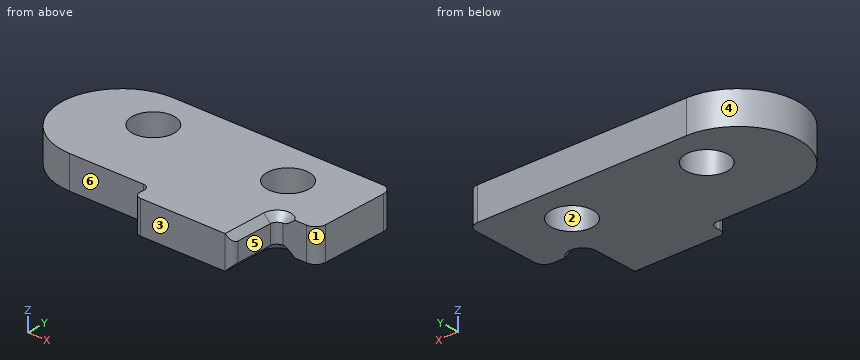
```python
from build123d import *

# Parameters (mm, degrees)
CROQUIS1_R                       = 6.125
SALIENTE_EXTRUIR1_DEPTH          = 9.53
BRIDA_DE_ARISTA1_STRIP_W         = 57.18
BRIDA_DE_ARISTA1_STRIP_H         = 9.53
BRIDA_DE_ARISTA1_STRIP_CUT_DEPTH = 85
BRIDA_DE_ARISTA1_DEPTH           = 85
REDONDEO1_R                      = 10
CHAFL_N1_SIZE                    = 25
CHAFL_N1_SIZE2                   = 20
REDONDEO2_R                      = 20
CORTAR_EXTRUIR3_DEPTH            = 148.009594705
CORTAR_EXTRUIR3_DEPTH_BACK       = 148.009594705
CROQUIS7_W                       = 70
CROQUIS7_H                       = 50
CORTAR_EXTRUIR5_DEPTH            = 92.169188443
CORTAR_EXTRUIR5_DEPTH_BACK       = 92.169188443
CROQUIS8_W                       = 21.963248134
CROQUIS8_H                       = 19.06
CORTAR_EXTRUIR6_REACH            = 68.882
CROQUIS10_W                      = 12
CROQUIS10_H                      = 15
SALIENTE_EXTRUIR3_START          = -9.53
SALIENTE_EXTRUIR3_DEPTH          = 9.53
REDONDEO3_R                      = 3
REDONDEO4_R                      = 2
CHAFL_N2_SIZE                    = 2


# Sheet-metal steps are written as plain solids
with BuildPart() as part:
    # Croquis1 → Saliente-Extruir1 (new body)
    with BuildSketch(Plane.XY):
        with BuildLine():
            Line((-5, 12.5), (59.758688568, 12.5))
            ThreePointArc((59.758688568, 12.5), (63.068757982, 11.936283192), (66.005639043, 10.308688094))
            Line((66.005639043, 10.308688094), (70.527359279, 6.691311906))
            ThreePointArc((70.527359279, 6.691311906), (73.464240341, 5.063716808), (76.774309755, 4.5))
            Line((76.774309755, 4.5), (123.266499161, 4.5))
            ThreePointArc((123.266499161, 4.5), (125.848488059, 3.781744193), (127.688665549, 1.833333333))
            ThreePointArc((127.688665549, 1.833333333), (129.41356885, -2.692366017), (130, -7.5))
            Line((130, -7.5), (130, -37.5))
            Line((130, -37.5), (45, -37.5))
            Line((45, -37.5), (45, -22.5))
            Line((45, -22.5), (-5, -22.5))
            ThreePointArc((-5, -22.5), (-22.5, -5), (-5, 12.5))
        make_face()
        Circle(CROQUIS1_R, mode=Mode.SUBTRACT)
        with Locations((40, 0)):
            Circle(CROQUIS1_R, mode=Mode.SUBTRACT)
    extrude(amount=SALIENTE_EXTRUIR1_DEPTH)

    # Brida de arista1 strip (across the edge) → Brida de arista1 strip cut (cut)
    with BuildSketch(Plane(origin=(45, -37.5, 9.53), x_dir=(0, 1, 0), z_dir=(1, 0, 0))):
        with Locations((-19.06, -4.765)):
            Rectangle(BRIDA_DE_ARISTA1_STRIP_W, BRIDA_DE_ARISTA1_STRIP_H)
    extrude(amount=BRIDA_DE_ARISTA1_STRIP_CUT_DEPTH, mode=Mode.SUBTRACT)

    # Brida de arista1 section (across the edge) → Brida de arista1 (add)
    with BuildSketch(Plane(origin=(45, -37.5, 9.53), x_dir=(0, 1, 0), z_dir=(1, 0, 0))):
        with BuildLine():
            Line((-9.53, 9.53), (-9.53, 40.47))
            Line((-9.53, 40.47), (0, 40.47))
            Line((0, 40.47), (0, 9.53))
            ThreePointArc((0, 9.53), (2.791272375, 2.791272375), (9.53, 0))
            Line((9.53, 0), (9.53, -9.53))
            ThreePointArc((9.53, -9.53), (-3.947455249, -3.947455249), (-9.53, 9.53))
        make_face()
    extrude(amount=BRIDA_DE_ARISTA1_DEPTH)

    # Redondeo1
    redondeo1_edges = [part.edges().sort_by_distance(p)[0] for p in [
        (45, -22.5, 4.765),
        (45, -42.265, 50),
    ]]
    fillet(redondeo1_edges, radius=REDONDEO1_R)

    # Chaflán1
    chafl_n1_edges = [part.edges().sort_by_distance(p)[0] for p in [
        (130, -42.265, 50),
    ]]
    chafl_n1_side = [part.faces().sort_by_distance(p)[0] for p in [
        (130, -17.735, 0.637386923),
    ]]
    chamfer(chafl_n1_edges, length=CHAFL_N1_SIZE, length2=CHAFL_N1_SIZE2, reference=chafl_n1_side[0])

    # Redondeo2
    redondeo2_edges = [part.edges().sort_by_distance(p)[0] for p in [
        (110, -42.265, 50),
        (130, -42.265, 25),
    ]]
    fillet(redondeo2_edges, radius=REDONDEO2_R)

    # Croquis7 → Cortar-Extruir3 (cut, two sides: drawn at the far end of the back side and taken through both)
    with BuildSketch(Plane(origin=(0, 0, 0), x_dir=(1, 0, 0), z_dir=(0, 1, 0)).offset(-CORTAR_EXTRUIR3_DEPTH_BACK)):
        with Locations((95, -25)):
            Rectangle(CROQUIS7_W, CROQUIS7_H)
    extrude(amount=CORTAR_EXTRUIR3_DEPTH + CORTAR_EXTRUIR3_DEPTH_BACK, mode=Mode.SUBTRACT)

    # Croquis8 → Cortar-Extruir5 (cut, two sides: drawn at the far end of the back side and taken through both)
    with BuildSketch(Plane.XY.offset(-CORTAR_EXTRUIR5_DEPTH_BACK)):
        with Locations((49.018375933, -37.5)):
            Rectangle(CROQUIS8_W, CROQUIS8_H)
    extrude(amount=CORTAR_EXTRUIR5_DEPTH + CORTAR_EXTRUIR5_DEPTH_BACK, mode=Mode.SUBTRACT)

    # Croquis10 → Cortar-Extruir6 (cut, up to next)
    with BuildSketch(Plane(origin=(0, 0, 0), x_dir=(-1, 0, 0), z_dir=(0, 0, -1)), mode=Mode.PRIVATE) as cortar_extruir6_sk1:
        with Locations((-54, -20.47)):
            Rectangle(CROQUIS10_W, CROQUIS10_H)
    cortar_extruir6_tool1 = extrude(cortar_extruir6_sk1.sketch, amount=-CORTAR_EXTRUIR6_REACH, mode=Mode.PRIVATE) & part.part
    add(cortar_extruir6_tool1.solids().sort_by_distance((54, -20.47, 0))[0], mode=Mode.SUBTRACT)

    # Croquis9 → Saliente-Extruir3 (add)
    with BuildSketch(Plane(origin=(0, 0, 0), x_dir=(-1, 0, 0), z_dir=(0, 0, -1)).offset(SALIENTE_EXTRUIR3_START)):
        with BuildLine():
            Line((-18.915105159, -22.5), (-35, -22.5))
            ThreePointArc((-35, -22.5), (-40.229722746, -23.976503065), (-43.915105159, -27.97))
            Line((-43.915105159, -27.97), (-18.915105159, -27.97))
            Line((-18.915105159, -27.97), (-18.915105159, -22.5))
        make_face()
    extrude(amount=SALIENTE_EXTRUIR3_DEPTH)

    # Redondeo3
    redondeo3_edges = [part.edges().sort_by_distance(p)[0] for p in [
        (60, -12.97, 4.765),
        (60, 12.497088016, 4.765),
    ]]
    fillet(redondeo3_edges, radius=REDONDEO3_R)

    # Redondeo4
    redondeo4_edges = [part.edges().sort_by_distance(p)[0] for p in [
        (48, -12.97, 4.765),
        (48, -27.97, 4.765),
        (18.915105159, -27.97, 4.765),
        (18.915105159, -22.5, 4.765),
    ]]
    fillet(redondeo4_edges, radius=REDONDEO4_R)

    # Chaflán2
    # the kernel refuses this chamfer: 2 mm, written as the material it takes off along each edge
    with BuildSketch(Plane(origin=(48, -31.113365976, 0), x_dir=(0.02749587661058563, 0, 0.9996219169112968), z_dir=(0, 1, 0))) as chafl_n2_piece_1:
        Polygon((CHAFL_N2_SIZE * 0.999621916911, -CHAFL_N2_SIZE * 0.0274958766106), (-CHAFL_N2_SIZE * 0.0274958766106, -CHAFL_N2_SIZE * 0.999621916911), (0, 0), align=None)
    extrude(amount=16.143365976, mode=Mode.SUBTRACT)
    with BuildSketch(Plane(origin=(48, -14.97, 9.53), x_dir=(-0.9996219169112968, 0, 0.02749587661058651), z_dir=(0, -1, 0))) as chafl_n2_piece_2:
        Polygon((CHAFL_N2_SIZE * 0.999621916911, CHAFL_N2_SIZE * 0.0274958766106), (-CHAFL_N2_SIZE * 0.0274958766106, CHAFL_N2_SIZE * 0.999621916911), (0, 0), align=None)
    extrude(amount=16.143365976, mode=Mode.SUBTRACT)
    with BuildSketch(Plane(origin=(50, -14.97, 0), x_dir=(0.5386859165215014, -0.8425066666450718, 0), z_dir=(-0.8425066666450718, -0.5386859165215014, 0))) as chafl_n2_piece_3:
        Polygon((2, CHAFL_N2_SIZE), (2 + CHAFL_N2_SIZE, 0), (2, 0), align=None)
    revolve(axis=Axis((50, -14.97, 0), (0, 0, 1)), revolution_arc=237.405771779, mode=Mode.SUBTRACT)
    with BuildSketch(Plane(origin=(50, -14.97, 9.53), x_dir=(0.5386859165215014, -0.8425066666450718, 0), z_dir=(-0.8425066666450718, -0.5386859165215014, 0))) as chafl_n2_piece_4:
        Polygon((2 + CHAFL_N2_SIZE, 0), (2, -CHAFL_N2_SIZE), (2, 0), align=None)
    revolve(axis=Axis((50, -14.97, 9.53), (0, 0, 1)), revolution_arc=237.405771779, mode=Mode.SUBTRACT)


solid = part.part
```
Here's how the part is built. I have some questions about the finished solid (model axes, mm). Face numbers are marked on the shaded views. A direction names the side the tool comes from. Coordinates: 2 decimals unless noted, no trailing zeros. Order: outer loops, then holes, each group sorted by start corner. A loop starts at its lowest first (then second) coordinate and runs counter-clockwise, first axis right, second up. Notation, with made-up numbers: (57.5, 45) - (112.5, 45) arc R15 ccw to (112.5, 60) - close; hole circle Ø8 at (-33.75, 76). An arc over 180 degrees is marked (long way). One line per question, with ' | ' between items. Start each with the question number.
1. If we section it at A-A (x = 0): Write out the boundary of the cut face in (y, z) (3 decimals).
2. If we mould it in two halves opening along X, with no side actions, what happens to the marked faces 1, 2 and 3? For each: released by +X, released by -X, zero draft, split by the parting line, or undercut.
3. Which directions (+Z, -Z, +X, -X, +Y, -Y) give clear straight access to the entire face, cutting with the end or side of a thin tool? Please do the marked faces 4, 5 and 6.
4. I'm going to push flat-ended pins straight in: pin 1 Ø1.2 at (y, z) = (-25.5, 6.5) entering from -X; pin 2 Ø1 at (x, z) = (15.5, 1.5) entering from -Y; pin 3 Ø1.5 at (y, z) = (-12, 3) entering from +X; pin 4 Ø7.5 at (x, y) = (40, 0) entering from +Z. Where does each tip first touch, or does it pass through?
5. If we section it at C-C (x = 40): Write out the boundary of the cut face in (y, z) (3 decimals).
6. If we section it at B-B (y = -3): Write out the boundary of the cut face in (x, z), and give its area (3 significant figures).
7. Please list where these lines run through material, in increasing order: line 1 along Y through (x, z) = (0, 6.5) (3 decimals); line 2 along Y through (x, z) = (40, 6) (3 decimals); line 3 along Y through (x, z) = (54, 2.5). Write a range as [from, to].
8. If we section it at D-D (z = 5.5): Give the number of separate pieces and of enclosed holes in the cut face, and give its area (3 significant figures).
Model answer:
1) outline: (-22.5, 0) - (-6.125, 0) - (-6.125, 9.53) - (-22.5, 9.53) - close; (6.125, 0) - (12.5, 0) - (12.5, 9.53) - (6.125, 9.53) - close
2) face 1: released by +X | face 2: undercut | face 3: zero draft
3) face 4: +Z, -Z, -X | face 5: +Z, -Z, +X, -Y | face 6: +Z, -Z, -X, -Y
4) pin 1: stops at x = 18.92 | pin 2: stops at y = -22.5 | pin 3: stops at x = 59.71 | pin 4: passes through
5) outline: (-27.97, 0) - (-6.125, 0) - (-6.125, 9.53) - (-27.97, 9.53) - close; (6.125, 0) - (12.5, 0) - (12.5, 9.53) - (6.125, 9.53) - close
6) outline: (-22.39, 0) - (-5.34, 0) - (-5.34, 9.53) - (-22.39, 9.53) - close; (5.34, 0) - (34.66, 0) - (34.66, 9.53) - (5.34, 9.53) - close; (45.34, 0) - (60, 0) - (60, 9.53) - (45.34, 9.53) - close | area: 582 mm²
7) line 1: y = [-22.5, -6.125], [6.125, 12.5] | line 2: y = [-27.97, -6.125], [6.125, 12.5] | line 3: y = [-12.97, 12.5]
8) separate pieces: 1 | enclosed holes: 2 | area: 2,560 mm²
